Design review of the part built by this model. Coordinates are the model's own, in mm. A direction names the side the tool comes from. Coordinates: 2 decimals unless noted, no trailing zeros. Loops run counter-clockwise (first coordinate to the right, second up) from the corner with the lowest first, then second, coordinate; pieces in that order, holes last. Notation, with made-up numbers: (47.5, 56) - (103.5, 56) arc R20 cw to (103.5, 82) - close; hole circle Ø8 at (24.5, 19). An arc over 180 degrees is marked (long way). Use one line per item in the form item = value. Start each with the question number.
(1) Tool access review of faces 1 (the face through (15.8, 18.5, -3.5)), 2 (the face through (0, 23, -10)), 3 (the face through (15.7, 18.5, 3.5)), 4 (the face through (-15.7, 18.5, -3.5)), 5 (the face through (0, 17, 16)): name each direction out of +Z, -Z, +X, -X, +Y, -Y from which nothing blocks a thin tool from reaching the whole face with its end or side.
(2) For L1, parallel to X at y = 18.3, z = 0; L2, parallel to Y at x = -4.5, z = -5; L3, parallel to X at y = 15, z = 0, list the stretches that pass through material, from the lowest coordinate up.
(3) Clearance check with flat-ended pins moving along their axes: pin 1 Ø1.1 at (x, y) = (-16.5, 18.5) entering from -Z; pin 2 Ø2 at (x, z) = (1, 16) entering from +Y; pin 3 Ø0.8 at (x, y) = (1.5, 16) entering from +Z. State where each tip first meets the part, or that it passes through.
(4) Add section B-B (z = 0). State the section outline as (x, y) points, plus the area to 3 significant figures.
(5) Add section A-A (x = 17.5). State the section outline as (y, z) points.
(6) The part is to be moulded in two halves that separate along Y. For faces 6 (the face through (-2, 21, -6)), 7 (the face through (0, 16, 15)), 8 (the face through (-20.14, 18.51, 2.6)), say which applies: pulls with the +Y half, pulls with the -Y half, needs draft (parallel to the pull), parting line crosses it, or undercut.
(7) Add section D-D (x = 0). State the section outline as (y, z) points, plus the area to 3 significant figures.
(8) Add section C-C (y = 16.25). State the section outline as (x, z) points, plus the area to 3 significant figures.
```python
from build123d import *

# Parameters (mm, degrees)
SKETCH_1_R          = 14
EXTRUDE_1_DEPTH     = 19
SKETCH_2_R          = 2
EXTRUDE_2_DEPTH     = 1
EXTRUDE_3_DEPTH     = 17
SKETCH_6_R          = 4.5
EXTRUDE_4_DEPTH     = 2
SKETCH_7_R          = 2.5
EXTRUDE_6_DEPTH     = 2
EXTRUDE_8_DEPTH     = 6
CUT_EXTRUDE_1_DEPTH = 2
CHAMFER_4_SIZE      = 0.3
FILLET_3_R          = 0.5
FILLET_4_R          = 0.5


with BuildPart() as part:
    # Эскиз1 → Бобышка-Вытянуть1 (new body)
    with BuildSketch(Plane(origin=(0, 0, 0), x_dir=(1, 0, 0), z_dir=(0, 1, 0))):
        with Locations(Location((0, 0, 0), (0, 0, 270))):
            Circle(SKETCH_1_R)
    extrude(amount=EXTRUDE_1_DEPTH)

    # Эскиз2 → Бобышка-Вытянуть2 (add)
    with BuildSketch(Plane(origin=(0, 19, 0), x_dir=(1, 0, 0), z_dir=(0, 1, 0))):
        with BuildLine():
            ThreePointArc((14, 0), (13.888415748, -1.764060095), (13.555441712, -3.5))
            Line((13.555441712, -3.5), (18, -3.5))
            ThreePointArc((18, -3.5), (20.121320344, -2.621320344), (21, -0.5))
            Line((21, -0.5), (21, 0.5))
            ThreePointArc((21, 0.5), (20.121320344, 2.621320344), (18, 3.5))
            Line((18, 3.5), (13.555441712, 3.5))
            ThreePointArc((13.555441712, 3.5), (13.888415748, 1.764060095), (14, 0))
        make_face()
        with Locations(Location((17.5, 0, 0), (0, 0, 270))):
            Circle(SKETCH_2_R, mode=Mode.SUBTRACT)
        with BuildLine():
            ThreePointArc((-21, -0.5), (-20.121320344, -2.621320344), (-18, -3.5))
            Line((-18, -3.5), (-13.555441712, -3.5))
            ThreePointArc((-13.555441712, -3.5), (-14, 0), (-13.555441712, 3.5))
            Line((-13.555441712, 3.5), (-18, 3.5))
            ThreePointArc((-18, 3.5), (-20.121320344, 2.621320344), (-21, 0.5))
            Line((-21, 0.5), (-21, -0.5))
        make_face()
        with Locations(Location((-17.5, 0, 0), (0, 0, 270))):
            Circle(SKETCH_2_R, mode=Mode.SUBTRACT)
    extrude(amount=-EXTRUDE_2_DEPTH)

    # Эскиз5 → Бобышка-Вытянуть3 (add)
    with BuildSketch(Plane(origin=(0, 19, 0), x_dir=(1, 0, 0), z_dir=(0, 1, 0))):
        with BuildLine():
            Line((-7.25, -17), (7.25, -17))
            Line((7.25, -17), (7.25, -11.976539567))
            ThreePointArc((7.25, -11.976539567), (0, -14), (-7.25, -11.976539567))
            Line((-7.25, -11.976539567), (-7.25, -17))
        make_face()
    extrude(amount=-EXTRUDE_3_DEPTH)

    # Эскиз6 → Бобышка-Вытянуть4 (add)
    with BuildSketch(Plane(origin=(0, 19, 0), x_dir=(1, 0, 0), z_dir=(0, 1, 0))):
        with Locations(Location((0, 8, 0), (0, 0, 270))):
            Circle(SKETCH_6_R)
    extrude(amount=EXTRUDE_4_DEPTH)

    # Эскиз7 → Бобышка-Вытянуть6 (add)
    with BuildSketch(Plane(origin=(0, 21, 0), x_dir=(1, 0, 0), z_dir=(0, 1, 0))):
        with Locations(Location((0, 8, 0), (0, 0, 270))):
            Circle(SKETCH_7_R)
    extrude(amount=EXTRUDE_6_DEPTH)

    # Эскиз9 → Бобышка-Вытянуть8 (add)
    with BuildSketch(Plane(origin=(0, 23, 0), x_dir=(1, 0, 0), z_dir=(0, 1, 0))):
        with BuildLine():
            Line((-2.053041545, 9.426541417), (2.053041545, 9.426541417))
            ThreePointArc((2.053041545, 9.426541417), (2.5, 8), (2.053041545, 6.573458583))
            Line((2.053041545, 6.573458583), (-2.053041545, 6.573458583))
            ThreePointArc((-2.053041545, 6.573458583), (-2.5, 8), (-2.053041545, 9.426541417))
        make_face()
    extrude(amount=EXTRUDE_8_DEPTH)

    # Эскиз11 → Вырез-Вытянуть1 (cut)
    with BuildSketch(Plane.XY.offset(17)):
        with BuildLine():
            Line((-2.75, 17), (2.75, 17))
            ThreePointArc((2.75, 17), (3.5, 16.25), (2.75, 15.5))
            Line((2.75, 15.5), (-2.75, 15.5))
            ThreePointArc((-2.75, 15.5), (-3.5, 16.25), (-2.75, 17))
        make_face()
    extrude(amount=-CUT_EXTRUDE_1_DEPTH, mode=Mode.SUBTRACT)

    # Фаска4
    chamfer_4_edges = [part.edges().sort_by_distance(p)[0] for p in [
        (2.5, 29, -8),
        (-2.5, 29, -8),
    ]]
    chamfer(chamfer_4_edges, length=CHAMFER_4_SIZE)

    # Скругление3
    fillet_3_edges = [part.edges().sort_by_distance(p)[0] for p in [
        (0, 2, 17),
        (7.25, 10.5, 17),
        (-7.25, 10.5, 17),
    ]]
    fillet(fillet_3_edges, radius=FILLET_3_R)

    # Скругление4
    fillet_4_edges = [part.edges().sort_by_distance(p)[0] for p in [
        (0, 0, -14),
    ]]
    fillet(fillet_4_edges, radius=FILLET_4_R)


solid = part.part
```
Computed values:
q1.face_1 = -Z, +X, +Y, -Y
q1.face_2 = -Z, +X, -X, +Y
q1.face_3 = +Z, +X, +Y, -Y
q1.face_4 = -Z, -X, +Y, -Y
q1.face_5 = +Z
q2.L1 = -21 to -19.5, -15.5 to 15.5, 19.5 to 21
q2.L2 = 0 to 19
q2.L3 = -14 to 14
q3.pin_1 = -3.5
q3.pin_2 = 19
q3.pin_3 = 15
q4.outline = (-21, 18) - (-19.5, 18) - (-19.5, 19) - (-21, 19) - close; (-15.5, 18) - (-14, 18) - (-14, 0.5) arc R0.5 ccw to (-13.5, 0) - (13.5, 0) arc R0.5 ccw to (14, 0.5) - (14, 18) - (15.5, 18) - (15.5, 19) - (-15.5, 19) - close; (19.5, 18) - (21, 18) - (21, 19) - (19.5, 19) - close
q4.area = 538 mm^2
q5.outline = (18, -3.5) - (19, -3.5) - (19, -2) - (18, -2) - close; (18, 2) - (19, 2) - (19, 3.5) - (18, 3.5) - close
q6.face_6 = pulls with the +Y half
q6.face_7 = undercut
q6.face_8 = needs draft
q7.outline = (0, -13.5) arc R0.5 ccw to (0.5, -14) - (19, -14) - (19, -12.5) - (21, -12.5) - (21, -10.5) - (23, -10.5) - (23, -9.43) - (29, -9.43) - (29, -6.57) - (23, -6.57) - (23, -5.5) - (21, -5.5) - (21, -3.5) - (19, -3.5) - (19, 17) - (17, 17) - (17, 15) - (15.5, 15) - (15.5, 17) - (2.5, 17) arc R0.5 ccw to (2, 16.5) - (2, 14) - (0.5, 14) arc R0.5 ccw to (0, 13.5) - close
q7.area = 625 mm^2
q8.outline = (-7.25, 11.98) arc R14 ccw (long way) to (7.25, 11.98) - (7.25, 16.5) arc R0.5 ccw to (6.75, 17) - (3.5, 17) - (3.5, 15) - (-3.5, 15) - (-3.5, 17) - (-6.75, 17) arc R0.5 ccw to (-7.25, 16.5) - close
q8.area = 655 mm^2
